```python
from build123d import *

# Parameters (mm, degrees)
F0_R     = 11
F1_DEPTH = 7
F2_W     = 29.0801070888
F2_H     = 28.3500068
F2_R     = 11
F2_R_2   = 9.4125034
F3_DEPTH = 1.5875
F4_R     = 1.7272
F5_DEPTH = 3.175


with BuildPart() as f1:
    # F0 (on Top) → F1 (new body)
    with BuildSketch(Plane.XY):
        Polygon((14.1750034, 14.1750034), (0, 14.1750034), (-14.9051036888, 14.1750034), (-14.9051036888, -14.1750034), (0, -14.1750034), (14.1750034, -14.1750034), align=None)
        Circle(F0_R, mode=Mode.SUBTRACT)
    extrude(amount=F1_DEPTH)

    # F2 (on face) → F3 (join)
    with BuildSketch(Plane.XY.offset(7)):
        with Locations((-0.3650501444, 0)):
            Rectangle(F2_W, F2_H)
        Circle(F2_R, mode=Mode.SUBTRACT)
        Circle(F2_R)
        Circle(F2_R_2, mode=Mode.SUBTRACT)
    extrude(amount=F3_DEPTH)

    # F4 (on face) → F5 (cut)
    with BuildSketch(Plane(origin=(-14.9051036888, 0, 0), x_dir=(0, -1, 0), z_dir=(-1, 0, 0))):
        with Locations((10.2062534, 3.96875)):
            Circle(F4_R)
        with Locations((-10.2062534, 3.96875)):
            Circle(F4_R)
    extrude(amount=-F5_DEPTH, mode=Mode.SUBTRACT)


solid = f1.part
```
Read the model definition and answer for the solid it produces. Units are mm, in the model's axes. A direction names the side the tool comes from. Coordinates: 2 decimals unless noted, no trailing zeros. Order: outer loops, then holes, each group sorted by start corner. A loop starts at its lowest first (then second) coordinate and runs counter-clockwise, first axis right, second up. Notation, with made-up numbers: (75, -1) - (96, -1) arc R20 ccw to (96, 10) - close; hole circle Ø8 at (47, 18.5). An arc over 180 degrees is marked (long way). Answer as a JSON object with one key per item and string values. Group by question number.
Item 1: A tool of negligible diameter and unlimited length cuts with its end or side. For faces 1 (the face through (-11.73, -10, 4)), 2 (the face through (-2.04, -9.19, 7.78)), from which of +Z, -Z, +X, -X, +Y, -Y can it reach the whole face along a straight path? Write none if from no direction.
Item 2: Consider probe 1 along Y at (x, z) = (-13, 4) (3 decimals); probe 2 along Y at (x, z) = (0, 7.5) (1 decimal); probe 3 along X at (y, z) = (3, 3) (3 decimals). Determine where each line is inside the solid, lowest interval first. Write a range as from..to.
Item 3: The mould has two halves that part along Z. Classify faces 3 (the face through (-2.38, -10.74, 3.45)), 4 (the face through (-7.03, 6.5, 8.588)), 5 (the face through (-4.94, 8.2, 7)), 6 (the face through (-13.34, 9.409, 2.436)): +Z half, -Z half, draft (parallel to the pull), parting line (faces both ways), or undercut.
Item 4: Section A-A (y = 0) is taken. Give the vertices of the cut face in (x, z) (1 decimal), plus the area to 3 significant figures.
Item 5: Section C-C (x = 0) is taken. Give the vertices of the cut face in (y, z) (1 decimal), plus the area to 3 significant figures.
Item 6: Flat-ended cylindrical pins translate along their axes: P1, Ø3, axis at y = -10.21, z = 3.97, coming from the -X side; P2, Ø6.5, axis at x = 5, y = -4.5, coming from the -Z side; P3, Ø3, axis at y = 10, z = 3.5, coming from the -X side. Find the tip coordinate at first contact, or state that the pin passes through.
Item 7: Section B-B (z = 0.5) is taken. Give the vertices of the cut face in (x, y) (3 decimals).
Item 8: Section D-D (x = -10) is taken. Give the vertices of the cut face in (y, z) (1 decimal), plus the area to 3 significant figures.
Results are:
{
 "1": {"face 1": "-X", "face 2": "+Z, -Z"},
 "2": {"probe 1": "y = -14.175..-11.933, -8.479..8.479, 11.933..14.175", "probe 2": "y = -14.2..-9.4, 9.4..14.2", "probe 3": "x = -14.905..-10.583, 10.583..14.175"},
 "3": {"face 3": "draft", "face 4": "+Z half", "face 5": "-Z half", "face 6": "undercut"},
 "4": {"outline": "(-14.9, 0) - (-11, 0) - (-11, 7) - (-9.4, 7) - (-9.4, 8.6) - (-14.9, 8.6) - close; (9.4, 7) - (11, 7) - (11, 0) - (14.2, 0) - (14.2, 8.6) - (9.4, 8.6) - close", "area": "65.8 mm^2"},
 "5": {"outline": "(-14.2, 0) - (-11, 0) - (-11, 7) - (-9.4, 7) - (-9.4, 8.6) - (-14.2, 8.6) - close; (9.4, 7) - (11, 7) - (11, 0) - (14.2, 0) - (14.2, 8.6) - (9.4, 8.6) - close", "area": "59.6 mm^2"},
 "6": {"P1": "stops at x = -11.73", "P2": "stops at z = 7", "P3": "stops at x = -14.91"},
 "7": {"outline": "(-14.905, -14.175) - (14.175, -14.175) - (14.175, 14.175) - (-14.905, 14.175) - close; hole circle Ø22 at (0, 0)"},
 "8": {"outline": "(-14.2, 0) - (-4.6, 0) - (-4.6, 7) - (4.6, 7) - (4.6, 0) - (14.2, 0) - (14.2, 8.6) - (-14.2, 8.6) - close", "area": "179 mm^2"}
}
